Part model, mm, in its own coordinate system. Face numbers are marked on the shaded views. A direction names the side the tool comes from. Coordinates: 2 decimals unless noted, no trailing zeros. Order: outer loops, then holes, each group sorted by start corner. A loop starts at its lowest first (then second) coordinate and runs counter-clockwise, first axis right, second up.
1) Pin check, flat tips, straight feed: pin 1 Ø6 at (y, z) = (8.5, 26) entering from +X; pin 2 Ø1.5 at (y, z) = (-1, 8) entering from -X; pin 3 Ø5.5 at (x, y) = (50.52, 0) entering from +Z. Stop position of each tip, or through.
2) Cut at D-D (y = -30.5). List the corners of the cut face in (x, z).
3) Cut at A-A (x = -11). List the corners of the cut face in (y, z), and give its area (3 significant figures).
4) Cut at B-B (z = -34.5). List the corners of the cut face in (x, y), and give its area (3 significant figures).
5) Tool access for the marked faces 1, 2 and 3: list every direction of +Z, -Z, +X, -X, +Y, -Y with a clear straight run to the whole face (end or side of a thin tool).
6) Wall check: L1, parallel to Y at x = 65, z = -42; L2, parallel to Z at x = 48.5, y = -3; L3, parallel to Z at x = 48, y = 33. Give the ranges that are in metal, low to high.
7) Cut at C-C (x = -65). List the corners of the cut face in (y, z), and give its area (4 significant figures).
```python
from build123d import *

# Parameters (mm, degrees)
SKETCH1_R                      = 40
BOSS_EXTRUDE1_DEPTH            = 39
CUT_EXTRUDE1_REACH             = 101.564
SKETCH2_W                      = 56
SKETCH2_H                      = 2
CUT_EXTRUDE1_DIRECTION_2_REACH = 101.564
CBORE_FOR_M6_SHCS1_AT_2_COUNT  = 2
CBORE_FOR_M6_SHCS1_AT_2_PITCH  = 22
CBORE_FOR_M6_SHCS1_AT_3_COUNT  = 2
CBORE_FOR_M6_SHCS1_AT_3_PITCH  = 44
CUT_EXTRUDE2_REACH             = 125.604
SKETCH5_R                      = 4.3
SKETCH5_R_2                    = 5.05


with BuildPart() as part:
    # Sketch1 → Boss-Extrude1 (new, symmetric)
    with BuildSketch(Plane(origin=(0, 0, 0), x_dir=(1, 0, 0), z_dir=(0, 1, 0))):
        with BuildLine():
            Line((-74, 54), (74, 54))
            Line((74, 54), (74, 39))
            Line((74, 39), (56, 39))
            Line((56, 39), (56, -26))
            Line((56, -26), (45.033320997, -26))
            ThreePointArc((45.033320997, -26), (0, -52), (-45.033320997, -26))
            Line((-45.033320997, -26), (-56, -26))
            Line((-56, -26), (-56, 39))
            Line((-56, 39), (-74, 39))
            Line((-74, 39), (-74, 54))
        make_face()
        with Locations(Location((0, 0, 0), (0, 0, 270))):
            Circle(SKETCH1_R, mode=Mode.SUBTRACT)
    extrude(amount=BOSS_EXTRUDE1_DEPTH, both=True)

    # Sketch2 → Cut-Extrude1 (cut, up to next)
    with BuildSketch(Plane(origin=(0, 0, 0), x_dir=(1, 0, 0), z_dir=(0, 1, 0)), mode=Mode.PRIVATE) as cut_extrude1_sk1:
        with Locations((28, 0)):
            Rectangle(SKETCH2_W, SKETCH2_H)
    cut_extrude1_tool1 = extrude(cut_extrude1_sk1.sketch, amount=-CUT_EXTRUDE1_REACH, mode=Mode.PRIVATE) & part.part
    add(cut_extrude1_tool1.solids().sort_by_distance((28, 0, 0))[0], mode=Mode.SUBTRACT)

    # Sketch2 → Cut-Extrude1 direction 2 (cut, up to next)
    with BuildSketch(Plane(origin=(0, 0, 0), x_dir=(1, 0, 0), z_dir=(0, 1, 0)), mode=Mode.PRIVATE) as cut_extrude1_direction_2_sk1:
        with Locations((28, 0)):
            Rectangle(SKETCH2_W, SKETCH2_H)
    cut_extrude1_direction_2_tool1 = extrude(cut_extrude1_direction_2_sk1.sketch, amount=CUT_EXTRUDE1_DIRECTION_2_REACH, mode=Mode.PRIVATE) & part.part
    add(cut_extrude1_direction_2_tool1.solids().sort_by_distance((28, 0, 0))[0], mode=Mode.SUBTRACT)

    # Sketch4 → CBORE for M6 SHCS1 (revolve, cut)
    with BuildSketch(Plane(origin=(50.516660498, 22, 26), x_dir=(0, -1, 0), z_dir=(1, 0, 0))):
        Polygon((0, 0), (0, 25), (3.3, 25), (3.3, 6), (5.5, 6), (5.5, 0), align=None)
    cbore_for_m6_shcs1 = revolve(axis=Axis((50.516660498, 22, 32.35), (0, 0, -1)), mode=Mode.SUBTRACT)

    # CBORE for M6 SHCS1 at 2: CBORE for M6 SHCS1 ×2
    with Locations(*[(0, -i * CBORE_FOR_M6_SHCS1_AT_2_PITCH, 0) for i in range(1, CBORE_FOR_M6_SHCS1_AT_2_COUNT)]):
        add(cbore_for_m6_shcs1, mode=Mode.SUBTRACT)

    # CBORE for M6 SHCS1 at 3: CBORE for M6 SHCS1 ×2
    with Locations(*[(0, -i * CBORE_FOR_M6_SHCS1_AT_3_PITCH, 0) for i in range(1, CBORE_FOR_M6_SHCS1_AT_3_COUNT)]):
        add(cbore_for_m6_shcs1, mode=Mode.SUBTRACT)

    # Sketch5 → Cut-Extrude2 (cut, up to next)
    with BuildSketch(Plane.XY.offset(-39), mode=Mode.PRIVATE) as cut_extrude2_sk1:
        with Locations((65, 22)):
            Circle(SKETCH5_R)
    cut_extrude2_tool1 = extrude(cut_extrude2_sk1.sketch, amount=-CUT_EXTRUDE2_REACH, mode=Mode.PRIVATE) & part.part
    # Sketch5 → Cut-Extrude2 (cut, up to next)
    with BuildSketch(Plane.XY.offset(-39), mode=Mode.PRIVATE) as cut_extrude2_sk2:
        with Locations((-65, -22)):
            Circle(SKETCH5_R)
    cut_extrude2_tool2 = extrude(cut_extrude2_sk2.sketch, amount=-CUT_EXTRUDE2_REACH, mode=Mode.PRIVATE) & part.part
    # Sketch5 → Cut-Extrude2 (cut, up to next)
    with BuildSketch(Plane.XY.offset(-39), mode=Mode.PRIVATE) as cut_extrude2_sk3:
        with Locations((-65, 22)):
            Circle(SKETCH5_R_2)
    cut_extrude2_tool3 = extrude(cut_extrude2_sk3.sketch, amount=-CUT_EXTRUDE2_REACH, mode=Mode.PRIVATE) & part.part
    # Sketch5 → Cut-Extrude2 (cut, up to next)
    with BuildSketch(Plane.XY.offset(-39), mode=Mode.PRIVATE) as cut_extrude2_sk4:
        with BuildLine():
            Line((65, -15.95), (74, -15.95))
            Line((74, -15.95), (74, -28.05))
            Line((74, -28.05), (65, -28.05))
            ThreePointArc((65, -28.05), (58.95, -22), (65, -15.95))
        make_face()
    cut_extrude2_tool4 = extrude(cut_extrude2_sk4.sketch, amount=-CUT_EXTRUDE2_REACH, mode=Mode.PRIVATE) & part.part
    add(cut_extrude2_tool1.solids().sort_by_distance((65, 22, -39))[0], mode=Mode.SUBTRACT)
    add(cut_extrude2_tool2.solids().sort_by_distance((-65, -22, -39))[0], mode=Mode.SUBTRACT)
    add(cut_extrude2_tool3.solids().sort_by_distance((-65, 22, -39))[0], mode=Mode.SUBTRACT)
    add(cut_extrude2_tool4.solids().sort_by_distance((67.057873, -22, -39))[0], mode=Mode.SUBTRACT)


solid = part.part
```
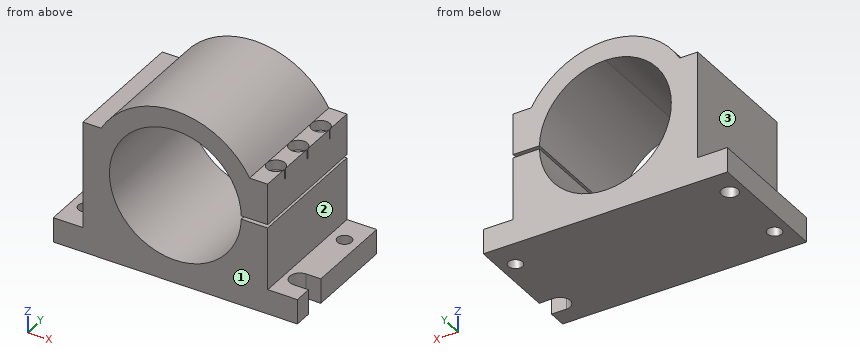
Geometry check:
1. pin 1: stops at x = 56
1. pin 2: stops at x = -56
1. pin 3: stops at z = -1
2. outline: (-74, -54) - (74, -54) - (74, -39) - (56, -39) - (56, -1) - (39.99, -1) arc R40 cw (long way) to (39.99, 1) - (56, 1) - (56, 26) - (45.03, 26) arc R52 ccw to (-45.03, 26) - (-56, 26) - (-56, -39) - (-74, -39) - close
3. outline: (-39, -54) - (39, -54) - (39, -38.46) - (-39, -38.46) - close; (-39, 38.46) - (39, 38.46) - (39, 50.82) - (-39, 50.82) - close
3. area: 2,180 mm2
4. outline: (-56, -39) - (-20.24, -39) - (-20.24, 39) - (-56, 39) - close; (20.24, -39) - (56, -39) - (56, 39) - (20.24, 39) - close
4. area: 5,580 mm2
5. face 1: +Z, -Z, +X, -X, -Y
5. face 2: +Z, +X, +Y, -Y
5. face 3: +Z, -X, +Y, -Y
6. L1: y = -39 to -28.05, -15.95 to 17.7, 26.3 to 39
6. L2: z = -54 to -1, 1 to 20
6. L3: z = -54 to -1, 1 to 26
7. outline: (-39, -54) - (-26.3, -54) - (-26.3, -39) - (-39, -39) - close; (-17.7, -54) - (16.95, -54) - (16.95, -39) - (-17.7, -39) - close; (27.05, -54) - (39, -54) - (39, -39) - (27.05, -39) - close
7. area: 889.5 mm2
